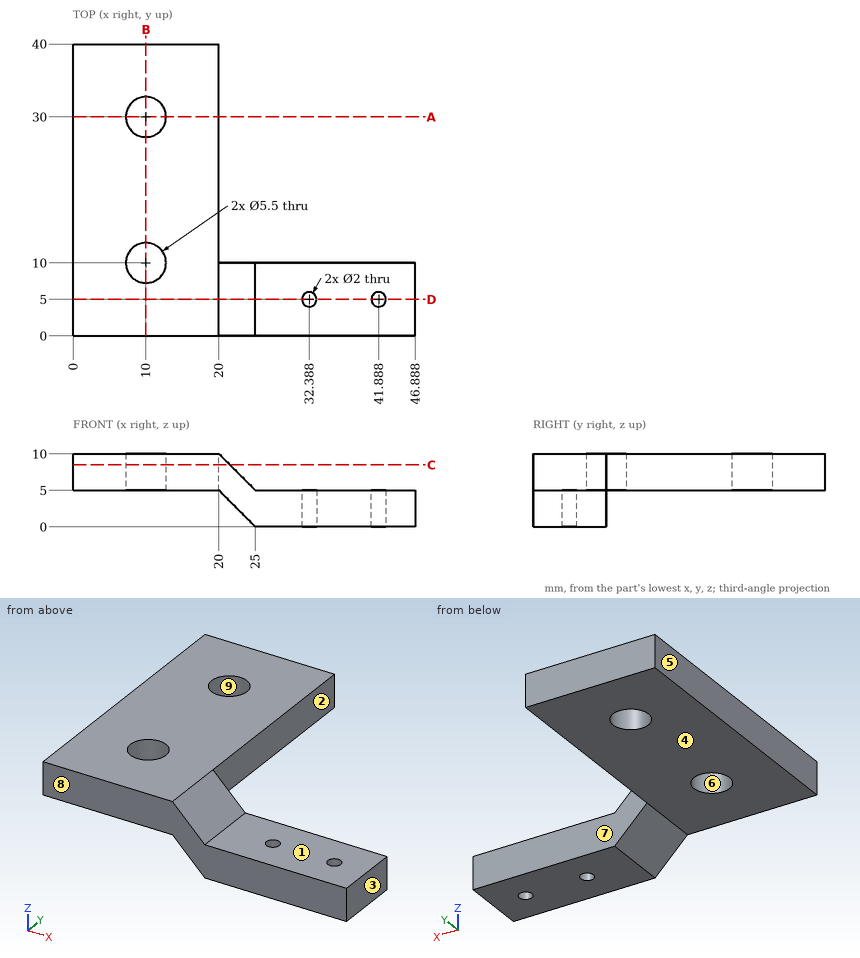
Part print with two shaded views. Sizes in mm from the minimum x, y, z corner. A direction names the side the tool comes from. Round coordinates to 2 decimals unless told otherwise and drop trailing zeros. Order: outer loops, then holes, each group sorted by start corner. A loop starts at its lowest first (then second) coordinate and runs counter-clockwise, first axis right, second up. Notation, with made-up numbers: M -36.5,4 L -29.5,4 A28 cw -29.5,43 Z; hole C 16,-36 d3. An arc over 180 degrees is marked long. Put each result on its own line as item: value. Start each with the question number.
1. Slice it at C-C on z = 8.5. List the corners of the cut face in (x, y).
2. Slice it at D-D on y = 5. List the corners of the cut face in (x, z).
3. Drill centre lines: probe 1 along Y at (x, z) = (10, 8.55); probe 2 along Y at (x, z) = (24.5, 3.25); probe 3 along X at (y, z) = (8, 6.25). Where is each one in solid material? Low to high. Write a range as [from, to].
4. Two-plate mould, pull along Y, no slides. Class the marked faces 6, 7, 8 and 9: +Y half, -Y half, draft (parallel to the pull), parting line (faces both ways), or undercut.
5. Drop flat-ended pins along their axis: pin 1 (5 mm diameter, centred on x = 10, y = 10, fed in from -Z); pin 2 (1 mm diameter, centred on x = 40, z = 2.5, fed in from +Y); pin 3 (3 mm diameter, centred on y = 35.5, z = 4, fed in from +X); pin 4 (6.5 mm diameter, centred on x = 10, y = 30, fed in from +Z). Give the stop position or say it passes through.
6. Tool access for the marked faces 1, 2, 3, 4 and 5: list every direction of +Z, -Z, +X, -X, +Y, -Y with a clear straight run to the whole face (end or side of a thin tool).
7. Slice it at A-A on y = 30. List the corners of the cut face in (x, z).
8. Slice it at B-B on x = 10. List the corners of the cut face in (y, z).
Findings:
1. outline: M 0,0 L 21.5,0 L 21.5,10 L 20,10 L 20,40 L 0,40 Z; hole C 10,10 d5.5; hole C 10,30 d5.5
2. outline: M 0,5 L 20,5 L 25,0 L 31.39,0 L 31.39,5 L 25,5 L 20,10 L 0,10 Z; M 33.39,0 L 40.89,0 L 40.89,5 L 33.39,5 Z; M 42.89,0 L 46.89,0 L 46.89,5 L 42.89,5 Z
3. probe 1: [0, 7.25], [12.75, 27.25], [32.75, 40]
3. probe 2: [0, 10]
3. probe 3: [0, 8.11], [11.89, 23.75]
4. face 6: undercut
4. face 7: +Y half
4. face 8: -Y half
4. face 9: undercut
5. pin 1: through
5. pin 2: y = 10
5. pin 3: x = 20
5. pin 4: z = 10
6. face 1: +Z, +X, +Y, -Y
6. face 2: +Z, -Z, +X, +Y
6. face 3: +Z, -Z, +X, +Y, -Y
6. face 4: -Z, -X, +Y, -Y
6. face 5: +Z, -Z, -X, +Y, -Y
7. outline: M 0,5 L 7.25,5 L 7.25,10 L 0,10 Z; M 12.75,5 L 20,5 L 20,10 L 12.75,10 Z
8. outline: M 0,5 L 7.25,5 L 7.25,10 L 0,10 Z; M 12.75,5 L 27.25,5 L 27.25,10 L 12.75,10 Z; M 32.75,5 L 40,5 L 40,10 L 32.75,10 Z
